Geometry: final body of the model. Coordinates: model frame, mm. Coordinates: 2 decimals unless noted, no trailing zeros. Write each loop counter-clockwise with the first axis right and the second up, starting at its lowest first coordinate (ties: lowest second). Pieces come first, ordered by that corner, then holes. Notation, with made-up numbers: (35, 83.25) - (44, 83.25) arc R16 cw to (44, 93.25) - close; hole circle Ø2 at (24, -10.75). An arc over 180 degrees is marked (long way). Answer as a JSON object with one key per item and string values. Group by question number.
Item 1: Section D-D on y = -33.5. Return loops of the section in (x, z), and give its area (4 significant figures).
Item 2: Line query: line 1 along Y through (x, z) = (-50, 3.75); line 2 along Y through (x, z) = (-23.5, 2); line 3 along X through (y, z) = (-11, 4.75). Output: solid intervals per line, ascending. Write a range as from..to.
Item 3: First-contact query: pin 1 Ø6 at (x, y) = (-23.5, 13.5) entering from +Z. Flat tip, straight axial feed; report the tip coordinate or a pass-through.
Item 4: Section B-B on x = -23.5. Return loops of the section in (y, z), and give its area (4 significant figures).
Item 5: Section A-A on y = 6. Return loops of the section in (x, z).
Item 6: Section C-C on z = 1.25. State how many separate pieces and enclosed holes the cut face has, and give its area (3 significant figures).
```python
from build123d import *

# Parameters (mm, degrees)
SKETCH1_W           = 120
SKETCH1_H           = 80
SKETCH1_R           = 2.5
SKETCH1_R_2         = 20
BOSS_EXTRUDE1_DEPTH = 6.35
FILLET1_R           = 2


with BuildPart() as part:
    # Sketch1 → Boss-Extrude1 (new body)
    with BuildSketch(Plane.XY):
        Rectangle(SKETCH1_W, SKETCH1_H)
        with Locations((-50, 30)):
            Circle(SKETCH1_R, mode=Mode.SUBTRACT)
        with Locations((-30, 30)):
            Circle(SKETCH1_R, mode=Mode.SUBTRACT)
        with Locations((-10, 30)):
            Circle(SKETCH1_R, mode=Mode.SUBTRACT)
        with Locations((10, 30)):
            Circle(SKETCH1_R, mode=Mode.SUBTRACT)
        with Locations((30, 30)):
            Circle(SKETCH1_R, mode=Mode.SUBTRACT)
        with Locations((50, 30)):
            Circle(SKETCH1_R, mode=Mode.SUBTRACT)
        with Locations((-50, 10)):
            Circle(SKETCH1_R, mode=Mode.SUBTRACT)
        with Locations((50, 10)):
            Circle(SKETCH1_R, mode=Mode.SUBTRACT)
        with Locations((0, -10)):
            Circle(SKETCH1_R_2, mode=Mode.SUBTRACT)
        with Locations((-23.5, 13.5)):
            Circle(SKETCH1_R, mode=Mode.SUBTRACT)
        with Locations((23.5, 13.5)):
            Circle(SKETCH1_R, mode=Mode.SUBTRACT)
        with Locations((23.5, -33.5)):
            Circle(SKETCH1_R, mode=Mode.SUBTRACT)
        with Locations((-23.5, -33.5)):
            Circle(SKETCH1_R, mode=Mode.SUBTRACT)
    extrude(amount=BOSS_EXTRUDE1_DEPTH)

    # Fillet1
    fillet1_edges = [part.edges().sort_by_distance(p)[0] for p in [
        (60, -40, 3.175),
        (-60, -40, 3.175),
        (-60, 40, 3.175),
        (60, 40, 3.175),
    ]]
    fillet(fillet1_edges, radius=FILLET1_R)


solid = part.part
```
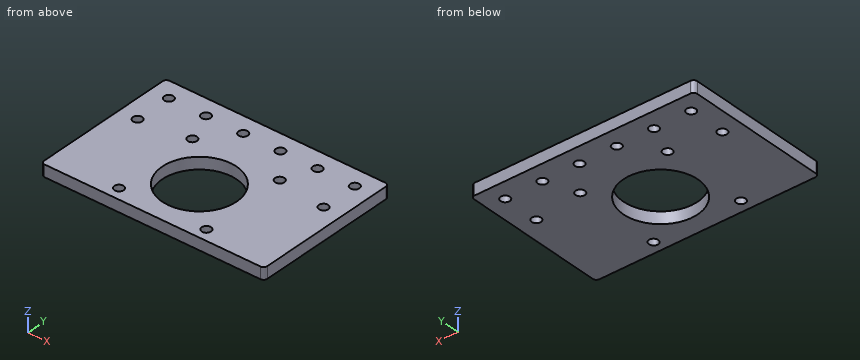
Checks:
{
 "1": {"outline": "(-60, 0) - (-26, 0) - (-26, 6.35) - (-60, 6.35) - close; (-21, 0) - (21, 0) - (21, 6.35) - (-21, 6.35) - close; (26, 0) - (60, 0) - (60, 6.35) - (26, 6.35) - close", "area": "698.5 mm^2"},
 "2": {"line 1": "-40..7.5, 12.5..27.5, 32.5..40", "line 2": "-40..-36, -31..11, 16..40", "line 3": "-60..-19.97, 19.97..60"},
 "3": {"pin 1": "z = 6.35"},
 "4": {"outline": "(-40, 0) - (-36, 0) - (-36, 6.35) - (-40, 6.35) - close; (-31, 0) - (11, 0) - (11, 6.35) - (-31, 6.35) - close; (16, 0) - (40, 0) - (40, 6.35) - (16, 6.35) - close", "area": "444.5 mm^2"},
 "5": {"outline": "(-60, 0) - (-12, 0) - (-12, 6.35) - (-60, 6.35) - close; (12, 0) - (60, 0) - (60, 6.35) - (12, 6.35) - close"},
 "6": {"separate pieces": "1", "enclosed holes": "13", "area": "8,100 mm^2"}
}
